Autodesk Inventor part; units mm, degrees
ref_plane "YZ Plane" through (0, 0, 0) normal (1, 0, 0) x (0, 1, 0)
ref_plane "XZ Plane" through (0, 0, 0) normal (0, 1, 0) x (-1, 0, 0)
ref_plane "XY Plane" through (0, 0, 0) normal (0, 0, 1) x (1, 0, 0)
sketch "Sketch1" plane through (0, 0, 0) normal (0, 1, 0) x (-1, 0, 0)
  line L0 (20.5, 16.2) -> (-20.5, 16.2)
  line L1 (-20.5, 16.2) -> (-20.5, -16.2)
  line L2 (-20.5, -16.2) -> (20.5, -16.2)
  line L3 (20.5, -16.2) -> (20.5, 16.2)
  point P0 (0, 0)
  dimension "d0" = 41
  dimension "d1" = 32.4
extrude "Extrusion1" add sketch "Sketch1" along normal blind 3
sketch "Sketch4" plane through (20.5, 0, -16.2) normal (0, 0, -1) x (-1, 0, 0)
  line L0 (41, 3) -> (0, 3)
  line L1 (0, 28.4) -> (41, 28.4)
  line L2 (0, 3) -> (21.5, 3)
  line L3 (21.5, 3) -> (21.5, 28.4)
  line L4 (21.5, 28.4) -> (0, 28.4)
  line L5 (0, 28.4) -> (0, 3)
  point P0 (20.5, 0)
  dimension "d12" = 21.5
extrude "Extrusion4" cut sketch "Sketch4" against normal blind 3
sketch "Sketch5" plane through (-20.5, 0, 16.2) normal (0, 0, 1) x (1, 0, 0)
  line L0 (41, 28.4) -> (0, 28.4)
  line L1 (41, 3) -> (0, 3)
  line L2 (0, 28.4) -> (21.5, 28.4)
  line L3 (21.5, 28.4) -> (21.5, 3)
  line L4 (21.5, 3) -> (0, 3)
  line L5 (0, 3) -> (0, 28.4)
  point P0 (20.5, 0)
  point P1 (19.5, 3)
  point P2 (19.5, 3)
  dimension "d15" = 21.5
extrude "Extrusion5" cut sketch "Sketch5" against normal blind 3
sketch "Sketch6" plane through (0, 3, 0) normal (0, 1, 0) x (1, 0, 0)
  circle A0 centre (13, 0) radius 4.25
  circle A1 centre (-13, 0) radius 4.25
  point P0 (0, 0)
  dimension "d20" = 8.5
  dimension "d21" = 8.5
extrude "Extrusion6" add sketch "Sketch6" along normal blind 3
sketch "Sketch7" plane through (0, 0, 0) normal (0, -1, 0) x (1, 0, 0)
  circle A0 centre (-13, 0) radius 4.25
  circle A1 centre (-13, 0) radius 2
  circle A2 centre (13, 0) radius 4.25
  circle A3 centre (13, 0) radius 2
  point P0 (0, 0)
  dimension "d24" = 4
  dimension "d25" = 4
extrude "Extrusion7" cut sketch "Sketch7" against normal blind 6 contours A1 | A3
sketch "Sketch8" plane through (0, 0, 0) normal (0, -1, 0) x (1, 0, 0)
  circle A0 centre (-13, 0) radius 2
  circle A1 centre (-13, 0) radius 3
  circle A2 centre (13, 0) radius 2
  circle A3 centre (13, 0) radius 3
  point P0 (0, 0)
  dimension "d28" = 6
  dimension "d29" = 6
extrude "Extrusion8" cut sketch "Sketch8" against normal blind 3 contours A0 | A1 | A2 | A3
sketch "Sketch16" plane through (0, 0, 0) normal (0, -1, 0) x (1, 0, 0)
  line L0 (-20.5, 16.2) -> (20.5, 16.2)
  line L1 (20.5, 16.2) -> (20.5, -16.2)
  line L2 (-20.5, 16.2) -> (20.5, 16.2)
  line L3 (20.5, 16.2) -> (20.5, 12.2)
  line L4 (20.5, 12.2) -> (-20.5, 12.2)
  line L5 (-20.5, 12.2) -> (-20.5, 16.2)
  point P0 (0, 0)
  point P1 (1, 16.2)
  point P2 (1, 16.2)
  dimension "d56" = 4
extrude "Extrusion15" cut sketch "Sketch16" against normal blind 50
sketch "Sketch17" plane through (0, 3, 0) normal (0, 1, 0) x (1, 0, 0)
  line L0 (20.5, 16.2) -> (-20.5, 16.2)
  line L1 (8, 16.2) -> (-8, 16.2)
  line L2 (-8, 16.2) -> (-8, 13.2)
  line L3 (-8, 13.2) -> (8, 13.2)
  line L4 (8, 13.2) -> (8, 16.2)
  point P0 (0, 0)
  dimension "d59" = 16
  dimension "d60" = 3
extrude "Extrusion16" add sketch "Sketch17" along normal blind 25.4
fillet "Fillet3" radius 1 8 edges at (0, 0, 12.2) (-20.5, 1.5, 12.2) (20.5, 1.5, 12.2) (20.5, 1.5, -16.2) (20.5, 0, -2) (-20.5, 0, -2) (-20.5, 1.5, -16.2) (0, 0, -16.2)
properties part number "zMount2"
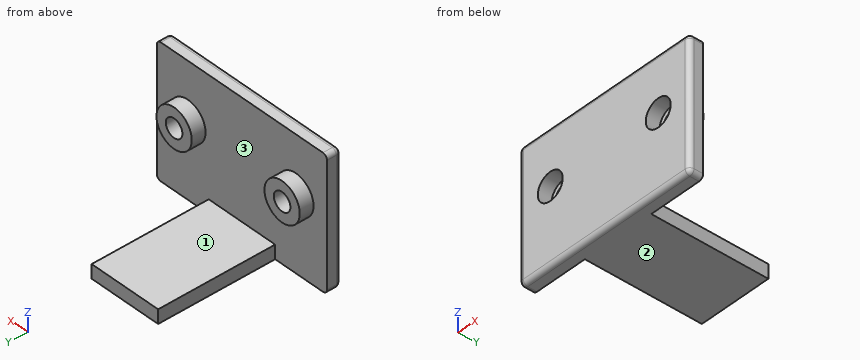
Build history of the part. All positions in model axes, mm. Face numbers are marked on the shaded views. A direction names the side the tool comes from. Round coordinates to 2 decimals unless told otherwise and drop trailing zeros. Write each loop counter-clockwise with the first axis right and the second up, starting at its lowest first coordinate (ties: lowest second). Pieces come first, ordered by that corner, then holes.
1) Band-saw the part on B-B, the plane z = 0. Give the number of separate pieces and of enclosed holes in the cut face, and give its area (3 significant figures).
2) Band-saw the part on D-D, the plane z = -9.75. List the corners of the cut face in (x, y), and give its area (3 significant figures).
3) Band-saw the part on A-A, the plane y = 4.5. List the corners of the cut face in (x, z).
4) Pin check, flat tips, straight feed: pin 1 (5 mm diameter, centred on x = 1.5, y = 8, fed in from +Z); pin 2 (6.5 mm diameter, centred on x = 13.5, z = -0.5, fed in from -Y); pin 3 (0.9 mm diameter, centred on y = 19.5, z = -14, fed in from +X); pin 4 (7 mm diameter, centred on x = -13, z = 0, fed in from +Y). Stop position of each tip, or through.
5) Band-saw the part on C-C, the plane x = -13. List the corners of the cut face in (y, z), and give its area (3 significant figures).
6) 3-axis set-ups, long thin cutter, end or side, ignore diameter. For the marked faces 1, 2 and 3: which of +Z, -Z, +X, -X, +Y, -Y reach the whole face in a straight line?
7) Drill centre lines: probe 1 along Z at (x, y) = (13, 5.3); probe 2 along Z at (x, y) = (13, 1.25); probe 3 along Y at (x, z) = (-12.5, 8.25). Where is each one in solid material? Low to high.
Ans:
1. separate pieces: 3
1. enclosed holes: 0
1. area: 114 mm2
2. outline: (-20.5, 1) arc R1 ccw to (-19.5, 0) - (19.5, 0) arc R1 ccw to (20.5, 1) - (20.5, 3) - (-20.5, 3) - close
2. area: 123 mm2
3. outline: circle Ø8.5 at (-13, 0); (-8, -16.2) - (8, -16.2) - (8, -13.2) - (-8, -13.2) - close; circle Ø8.5 at (13, 0); hole circle Ø4 at (-13, 0); hole circle Ø4 at (13, 0)
4. pin 1: stops at z = -13.2
4. pin 2: stops at y = 0
4. pin 3: stops at x = 8
4. pin 4: stops at y = 6
5. outline: (0, -15.2) arc R1 ccw to (1, -16.2) - (3, -16.2) - (3, -4.25) - (6, -4.25) - (6, -2) - (3, -2) - (3, -3) - (0, -3) - close; (0, 3) - (3, 3) - (3, 2) - (6, 2) - (6, 4.25) - (3, 4.25) - (3, 12.2) - (1, 12.2) arc R1 ccw to (0, 11.2) - close
5. area: 80.3 mm2
6. face 1: +Z, +X, -X, +Y
6. face 2: -Z, +X, -X, +Y, -Y
6. face 3: +Y
7. probe 1: z = -4.25 to -2, 2 to 4.25
7. probe 2: z = -16.2 to -3, 3 to 12.2
7. probe 3: y = 0 to 3
